Here's how the part is built. I have some questions about the finished solid (model axes, mm). Round coordinates to 2 decimals unless told otherwise and drop trailing zeros. Order: outer loops, then holes, each group sorted by start corner. A loop starts at its lowest first (then second) coordinate and runs counter-clockwise, first axis right, second up. Notation, with made-up numbers: (-2.75, 73.25) -> (12.25, 73.25) arc R25 cw to (12.25, 99.25) -> close; hole circle Ø1 at (16, -35.75). An arc over 180 degrees is marked (long way). Use a Markdown table: item, result. Add a question column.
(1) I want a section at A-A, the plane x = -13. Please give me the cut outline in (y, z).
(2) If I drill on probe 1 along Z at (x, y) = (-32.5, 0.25); probe 2 along Z at (x, y) = (-37.5, 3); probe 3 along Z at (x, y) = (-22, 1.9), over which ranges is the centre line in solid material (lowest first)?
(3) I want a section at D-D, the plane z = -117.5. Please give me the cut outline in (x, y), then the cut area to 3 significant figures.
(4) I want a section at C-C, the plane x = -7.5. Please give me the cut outline in (y, z), then the cut area to 3 significant figures.
(5) I want a section at B-B, the plane y = 2.85. Give the number of separate pieces and of enclosed holes in the cut face, then the cut area to 3 significant figures.
Autodesk Inventor part; units mm, degrees
ref_plane "YZ Plane" through (0, 0, 0) normal (1, 0, 0) x (0, 1, 0)
ref_plane "XZ Plane" through (0, 0, 0) normal (0, 1, 0) x (-1, 0, 0)
ref_plane "XY Plane" through (0, 0, 0) normal (0, 0, 1) x (1, 0, 0)
sketch "Sketch1" plane through (0, 0, 0) normal (0, 1, 0) x (-1, 0, 0)
  line L0 (0, 0) -> (45, 0)
  line L1 (45, 0) -> (45, -128)
  line L2 (45, -128) -> (0, -128)
  line L3 (0, -128) -> (0, 0)
  line L4 (37.5, -14) -> (7.5, -14) construction
  line L5 (7.5, -14) -> (7.5, -46) construction
  line L6 (7.5, -46) -> (37.5, -46) construction
  line L7 (37.5, -46) -> (37.5, -14) construction
  circle A0 centre (37.5, -46) radius 2.7
  circle A1 centre (37.5, -14) radius 2.7
  circle A2 centre (7.5, -14) radius 2.7
  circle A3 centre (7.5, -46) radius 2.7
  line L8 (22.5, -14) -> (22.5, 0) construction
  circle A4 centre (5, -107.5) radius 1.5
  circle A5 centre (40, -107.5) radius 1.5
  line L9 (40, -109) -> (5, -109)
  line L10 (5, -106) -> (40, -106)
  line L11 (21, -109) -> (21, -116)
  line L12 (24, -116) -> (24, -109)
  line L13 (22.5, -116) -> (22.5, -109) construction
  circle A6 centre (40, -117.5) radius 1.5
  line L14 (5, -116) -> (40, -116)
  line L15 (40, -119) -> (5, -119)
  circle A7 centre (5, -117.5) radius 1.5
  line L16 (17.5, -109) -> (17.5, -116)
  line L17 (27.5, -116) -> (27.5, -109)
  line L18 (22.5, -116) -> (22.5, -128) construction
  line L19 (21, -111.5) -> (24, -111.5)
  line L20 (24, -113.5) -> (21, -113.5)
  point P0 (25, -109)
  point P1 (25, -116)
  point P2 (15, -116)
  point P3 (15, -109)
  point P4 (21.5, -116)
  point P5 (18.5, -116)
  point P6 (22.5, -112.5)
  point P7 (22.5, -111.5)
  dimension "d0" = 128
  dimension "d1" = 45
  dimension "d2" = 30
  dimension "d3" = 32
  dimension "d4" = 5.4
  dimension "d5" = 14
  dimension "d6" = 3
  dimension "d7" = 35
  dimension "d8" = 7
  dimension "d9" = 3
  dimension "d10" = 35
  dimension "d11" = 5
  dimension "d12" = 5
  dimension "d13" = 12
  dimension "d16" = 3
  dimension "d17" = 1.5
  dimension "d18" = 2
  dimension "d19" = 1
extrude "Extrusion1" add sketch "Sketch1" along normal blind 4 contours L0 L1 L2 L3 | L9 L11 L14 L16 | L17 L14 L12 L9 | L19 L12 L20 L11
fillet "Fillet1" radius 1.5 4 edges at (-24, 2, -113.5) (-21, 2, -113.5) (-24, 2, -111.5) (-21, 2, -111.5)
equation "\"d12\" = d11"
equation "\"d17\" = 0.5 * d16"
properties part number "p2_3DPrint"
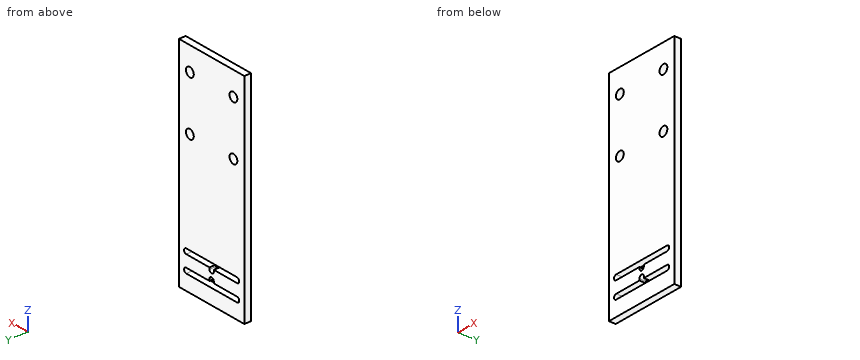
Taken from the geometry:
| question | item | result |
|---|---|---|
| 1 | outline | (0, -128) -> (4, -128) -> (4, -119) -> (0, -119) -> close; (0, -116) -> (4, -116) -> (4, -109) -> (0, -109) -> close; (0, -106) -> (4, -106) -> (4, 0) -> (0, 0) -> close |
| 2 | probe 1 | z = -128 to -119, -116 to -109, -106 to 0 |
| 2 | probe 2 | z = -128 to -119, -116 to -109, -106 to -48.7, -43.3 to -16.7, -11.3 to 0 |
| 2 | probe 3 | z = -128 to -119, -113.59 to -111.41, -106 to 0 |
| 3 | outline | (-45, 0) -> (-41.5, 0) -> (-41.5, 4) -> (-45, 4) -> close; (-3.5, 0) -> (0, 0) -> (0, 4) -> (-3.5, 4) -> close |
| 3 | area | 28.0 mm2 |
| 4 | outline | (0, -128) -> (4, -128) -> (4, -119) -> (0, -119) -> close; (0, -116) -> (4, -116) -> (4, -109) -> (0, -109) -> close; (0, -106) -> (4, -106) -> (4, -48.7) -> (0, -48.7) -> close; (0, -43.3) -> (4, -43.3) -> (4, -16.7) -> (0, -16.7) -> close; (0, -11.3) -> (4, -11.3) -> (4, 0) -> (0, 0) -> close |
| 4 | area | 445 mm2 |
| 5 | separate pieces | 1 |
| 5 | enclosed holes | 6 |
| 5 | area | 5,430 mm2 |
